Input: part model. Units: mm. Frame: model coordinates. A direction names the side the tool comes from. Round coordinates to 2 decimals unless told otherwise and drop trailing zeros. Loops run counter-clockwise (first coordinate to the right, second up) from the corner with the lowest first, then second, coordinate; pieces in that order, holes last. Notation, with made-up numbers: M 55,-1 L 63,-1 A14 cw 63,25 Z; hole C 81.25,42.25 d7. An arc over 180 degrees is marked long. Use one line per item in the form item = value. Start each with the question number.
Q1. Section query A-A, the plane x = 0. Output: boundary loops of the cut face in (y, z), and give its area (3 significant figures).
Q2. Section query C-C, the plane y = 8. Output: boundary loops of the cut face in (x, z).
Q3. Access query for faces 4 (the flat face through (-20, 4.6, -2.1)), 5 (the cylindrical face through (40.06, 12.62, -2.46)), 6 (the flat face through (-30.1, 2.3, -20)). Directions: +Z, -Z, +X, -X, +Y, -Y. A direction counts if a zero-diameter tool reaches every point of the face in a straight line with its end or side. Return the directions, or none.
Q4. Ray query, line 1 along Y through (x, z) = (0, -3.3); line 2 along Y through (x, z) = (30.5, -1.75); line 3 along X through (y, z) = (-4, -11.25). Return the intervals inside material, ascending.
Q5. First-contact query: P1, Ø4.5, axis at x = -24, z = -4, coming from the +Y side; P2, Ø8, axis at x = 19.5, y = 24.5, coming from the -Z side; P3, Ø8, axis at y = -34, z = -11.5, coming from the +X side; P4, Ø7.5, axis at x = -24, z = -11, coming from the +Y side. Flat tips, straight axial feed; report the tip coordinate or a pass-through.
Q6. Section query D-D, the plane z = 1.75. Output: boundary loops of the cut face in (x, y).
Q7. Mould query, pull axis Y, two halves, no side actions, for faces 1 (the flat face through (16, -39, -5)), 2 (the flat face through (-28, 2, -8)), 3 (the cylindrical face through (-9.538, -42.954, -2.465)). Classes: pulls with the +Y half, pulls with the -Y half, needs draft (parallel to the pull), parting line crosses it, or undercut.
Q8. Section query B-B, the plane z = -12.25. Output: boundary loops of the cut face in (x, y).
```python
from build123d import *

# Parameters (mm, degrees)
ESBO_O1_R                = 50
RESSALTO_EXTRUS_O1_DEPTH = 5
RESSALTO_EXTRUS_O2_START = -20
RESSALTO_EXTRUS_O2_DEPTH = 20
ESBO_O1_4_R              = 44
ESBO_O1_4_R_2            = 42
RESSALTO_EXTRUS_O3_DEPTH = 5


with BuildPart() as part:
    # Esbo_o1 → Ressalto-extrus_o1 (new body)
    with BuildSketch(Plane.XY):
        Circle(ESBO_O1_R)
        with BuildLine():
            ThreePointArc((35, 2), (37, 0), (35, -2))
            Line((35, -2), (20, -2))
            Line((20, -2), (20, -18))
            ThreePointArc((20, -18), (0, -38), (-20, -18))
            Line((-20, -18), (-20, -2))
            Line((-20, -2), (-35, -2))
            ThreePointArc((-35, -2), (-37, 0), (-35, 2))
            Line((-35, 2), (-20, 2))
            Line((-20, 2), (-20, 18))
            ThreePointArc((-20, 18), (0, 38), (20, 18))
            Line((20, 18), (20, 2))
            Line((20, 2), (35, 2))
        make_face(mode=Mode.SUBTRACT)
    extrude(amount=RESSALTO_EXTRUS_O1_DEPTH)

    # Esbo_o1_3 → Ressalto-extrus_o2 (add)
    with BuildSketch(Plane.XY.offset(RESSALTO_EXTRUS_O2_START)):
        with BuildLine():
            ThreePointArc((35, 2), (36.414213562, 1.414213562), (37, 0))
            Line((37, 0), (40, 0))
            ThreePointArc((40, 0), (38.535533906, 3.535533906), (35, 5))
            Line((35, 5), (20, 5))
            Line((20, 5), (20, 2))
            Line((20, 2), (35, 2))
        make_face()
        with BuildLine():
            Line((40, 0), (37, 0))
            ThreePointArc((37, 0), (36.414213562, -1.414213562), (35, -2))
            Line((35, -2), (20, -2))
            Line((20, -2), (20, -5))
            Line((20, -5), (35, -5))
            ThreePointArc((35, -5), (38.535533906, -3.535533906), (40, 0))
        make_face()
        with BuildLine():
            Line((-35, -5), (-20, -5))
            Line((-20, -5), (-20, -2))
            Line((-20, -2), (-35, -2))
            ThreePointArc((-35, -2), (-37, 0), (-35, 2))
            Line((-35, 2), (-20, 2))
            Line((-20, 2), (-20, 5))
            Line((-20, 5), (-35, 5))
            ThreePointArc((-35, 5), (-40, 0), (-35, -5))
        make_face()
    extrude(amount=RESSALTO_EXTRUS_O2_DEPTH)

    # Esbo_o1_4 → Ressalto-extrus_o3 (add)
    with BuildSketch(Plane.XY):
        Circle(ESBO_O1_4_R)
        Circle(ESBO_O1_4_R_2, mode=Mode.SUBTRACT)
    extrude(amount=-RESSALTO_EXTRUS_O3_DEPTH)


solid = part.part
```
Results found:
q1.outline = M -50,0 L -44,0 L -44,-5 L -42,-5 L -42,0 L -38,0 L -38,5 L -50,5 Z; M 38,0 L 42,0 L 42,-5 L 44,-5 L 44,0 L 50,0 L 50,5 L 38,5 Z
q1.area = 140 mm²
q2.outline = M -49.36,0 L -43.27,0 L -43.27,-5 L -41.23,-5 L -41.23,0 L -20,0 L -20,5 L -49.36,5 Z; M 20,0 L 41.23,0 L 41.23,-5 L 43.27,-5 L 43.27,0 L 49.36,0 L 49.36,5 L 20,5 Z
q3.face_4 = +Z, -Z
q3.face_5 = -Z
q3.face_6 = -Z, +X, -X, +Y, -Y
q4.line_1 = -44 to -42, 42 to 44
q4.line_2 = -31.71 to -28.87, -5 to -2, 2 to 5, 28.87 to 31.71
q4.line_3 = -38 to -20, 20 to 38
q5.P1 = 38.25
q5.P2 = 0
q5.P3 = through
q5.P4 = 5
q6.outline = C 0,0 d100; hole M -35,-2 L -20,-2 L -20,-18 A20 ccw 20,-18 L 20,-2 L 35,-2 A2 ccw 35,2 L 20,2 L 20,18 A20 ccw -20,18 L -20,2 L -35,2 A2 ccw Z
q7.face_1 = needs draft
q7.face_2 = undercut
q7.face_3 = parting line crosses it
q8.outline = M -35,-5 L -20,-5 L -20,-2 L -35,-2 A2 cw -35,2 L -20,2 L -20,5 L -35,5 A5 ccw Z; M 20,-5 L 35,-5 A5 ccw 35,5 L 20,5 L 20,2 L 35,2 A2 cw 35,-2 L 20,-2 Z
